from build123d import *

# Parameters (mm, degrees)
SFAZOWANIE1_SIZE = 1


with BuildPart() as part:
    # Szkic1 → Obrót1 (revolve)
    with BuildSketch(Plane.XY, mode=Mode.PRIVATE) as obr_t1_sk:
        Polygon((-17.5, 15), (-17.5, 7), (-3.5, 7), (-3.5, 2), (3.5, 2), (3.5, 7), (17.5, 7), (17.5, 15), (4, 15), (4, 14), (-4, 14), (-4, 15), align=None)
    revolve(obr_t1_sk.sketch.rotate(Axis((0, 0, 0), (1, 0, 0)), 90), axis=Axis((0, 0, 0), (1, 0, 0)))

    # Sfazowanie1
    sfazowanie1_edges = [part.edges().sort_by_distance(p)[0] for p in [
        (4, 0, -15),
        (17.5, 0, -15),
        (-17.5, 0, -15),
        (-4, 0, -15),
    ]]
    chamfer(sfazowanie1_edges, length=SFAZOWANIE1_SIZE - 0.0001)  # a hair under: the kernel refuses the full size


solid = part.part
Design review of the part built by this model. Coordinates are the model's own, in mm. A direction names the side the tool comes from. Coordinates: 2 decimals unless noted, no trailing zeros. Loops run counter-clockwise (first coordinate to the right, second up) from the corner with the lowest first, then second, coordinate; pieces in that order, holes last. Notation, with made-up numbers: M 89,34 L 109,34 A29 ccw 109,62 Z; hole C 61.25,-17 d9. An arc over 180 degrees is marked long. Answer as CSV lines item,"result".
Item 1: Add section D-D on x = 3. State the section outline as (y, z) points, plus the area to 3 significant figures.
Answer list:
outline,"C 0,0 d28; hole C 0,0 d4"
area,"603 mm²"
Item 2: Add section C-C on x = -9.5. State the section outline as (y, z) points, plus the area to 3 significant figures.
Answer list:
outline,"C 0,0 d30; hole C 0,0 d14"
area,"553 mm²"
Item 3: For P1, Ø5, axis at x = -8, y = 5.5, coming from the -Z side; P2, Ø5, axis at x = -1, z = -4, coming from the +Y side; P3, Ø5, axis at x = 3.5, z = -8, coming from the +Y side; P4, Ø3.5, axis at y = 0, z = 0, coming from the -X side, all flat-tipped, find the tip position at first contact; note any pin that passes through.
Answer list:
P1,"z = -14.7"
P2,"y = 13.92"
P3,"y = 13.75"
P4,"through"
Item 4: For probe 1 along Y at (x, z) = (9.5, 0); probe 2 along X at (y, z) = (2, -3.75); probe 3 along X at (y, z) = (-10.5, -10), list the stretches that pass through material, from the lowest coordinate up.
Answer list:
probe 1,"-15 to -7, 7 to 15"
probe 2,"-3.5 to 3.5"
probe 3,"-17 to -4.5, 4.5 to 17"
Item 5: Machinability: for faces 5 (the face through (10.67, -12.65, 8.06)), 6 (the face through (3.5, 1, 2)), 7 (the face through (-10.4, 6.21, 3.23)), which of the approach directions +Z, -Z, +X, -X, +Y, -Y give a long, thin tool a straight path to every point of the face, cutting with its end or side? Answer none if there is none.
Answer list:
face 5,"+X, -X"
face 6,"+X"
face 7,"-X"
Item 6: The part is to be moulded in two halves that separate along X. For faces 1 (the face through (-17.5, -6.4, -3.3)), 2 (the face through (-0.1, 12.4, 6.5)), 3 (the face through (10.6, 6.21, 3.23)), 4 (the face through (17.5, -3.3, 6.4)), say which applies: pulls with the +X half, pulls with the -X half, needs draft (parallel to the pull), parting line crosses it, or undercut.
Answer list:
face 1,"pulls with the -X half"
face 2,"undercut"
face 3,"needs draft"
face 4,"pulls with the +X half"
